Here's the drawing with two shaded views (mm, measured from the low corner). I have some questions. A direction names the side the tool comes from. Round coordinates to 2 decimals unless told otherwise and drop trailing zeros. Write each loop counter-clockwise with the first axis right and the second up, starting at its lowest first coordinate (ties: lowest second). Pieces come first, ordered by that corner, then holes. Notation, with made-up numbers: M 73.25,3.5 L 127.25,3.5 A34 ccw 127.25,33.5 Z; hole C 75,75.5 d3. An arc over 180 degrees is marked long. Answer as a JSON object with one key per item and string values. Group by question number.
1) Suppose I cut it at A-A, the plane x = 120. Write out the boundary of the cut face in (y, z), and give its area (3 significant figures).
2) Suppose I cut it at C-C, the plane z = 36. Write out the boundary of the cut face in (x, y).
3) I'm going to push flat-ended pins straight in: pin 1 Ø7.5 at (x, y) = (65.5, 120.5) entering from +Z (1 decimal); pin 2 Ø5 at (x, y) = (89.5, 3) entering from +Z; pin 3 Ø17 at (y, z) = (62.12, 48.86) entering from -X. Where does each tip first touch, or does it pass through?
4) If we mould it in two halves opening along X, with no side actions, what happens to the marked faces 3, 4 and 5? For each: +X half, -X half, draft (parallel to the pull), parting line (faces both ways), or undercut.
5) Suppose I cut it at D-D, the plane z = 52. Write out the boundary of the cut face in (x, y).
6) On a 3-axis mill with a long thin cutter (end or side, diameter ignored), from which of +Z, -Z, +X, -X, +Y, -Y can I reach the whole of each face in a straight line? I mean the marked faces 1 and 2. Say none if no direction works.
7) Please list where these lines run through material, in increasing order: L1, parallel to X at y = 51, z = 64; L2, parallel to Y at x = 46, z = 27.5; L3, parallel to X at y = 119, z = 82. Write a range as [from, to].
8) Suppose I cut it at B-B, the plane y = 84. Write out the boundary of the cut face in (x, z), and give its area (3 significant figures).
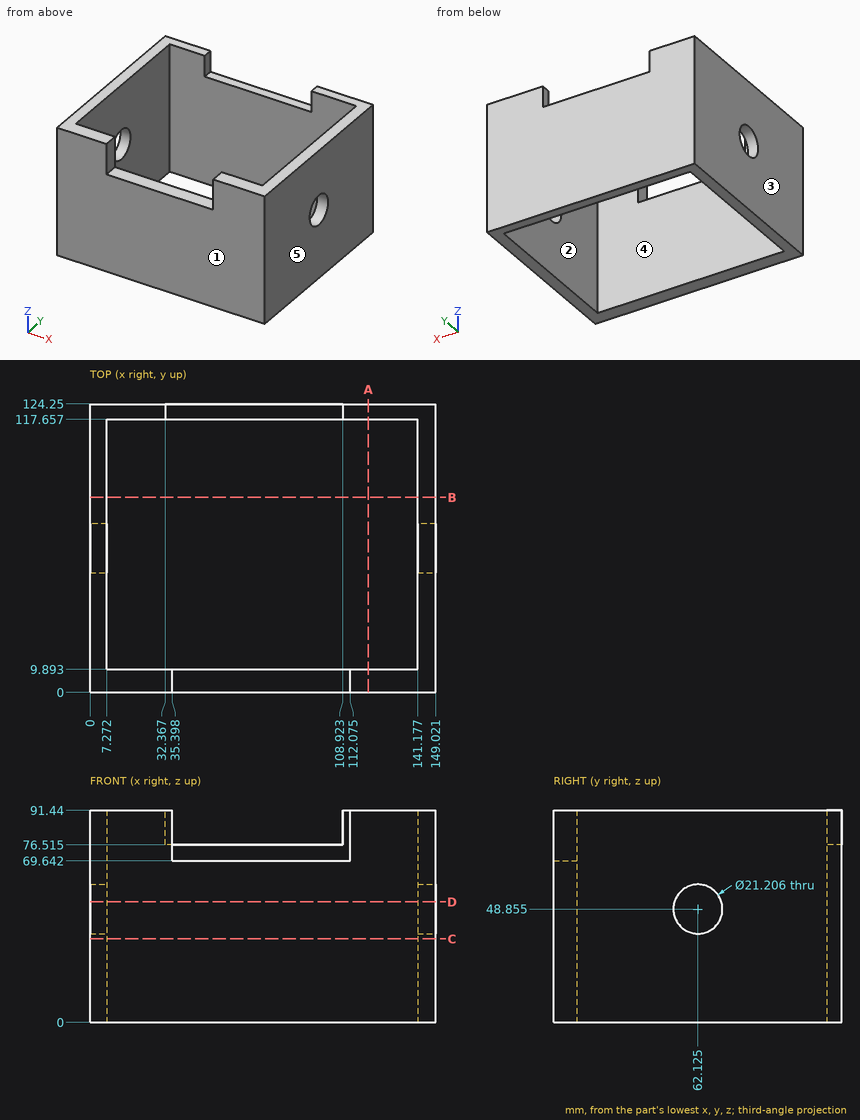
Results:
{
 "1": {"outline": "M 0,0 L 9.89,0 L 9.89,91.44 L 0,91.44 Z; M 117.66,0 L 124.25,0 L 124.25,91.44 L 117.66,91.44 Z", "area": "1,510 mm^2"},
 "2": {"outline": "M 0,0 L 149.02,0 L 149.02,124.25 L 0,124.25 Z; hole M 7.27,9.89 L 141.18,9.89 L 141.18,117.66 L 7.27,117.66 Z"},
 "3": {"pin 1": "z = 76.5", "pin 2": "z = 69.64", "pin 3": "through"},
 "4": {"face 3": "-X half", "face 4": "undercut", "face 5": "+X half"},
 "5": {"outline": "M 0,0 L 149.02,0 L 149.02,52 L 141.18,52 L 141.18,9.89 L 7.27,9.89 L 7.27,52 L 0,52 Z; M 0,72.25 L 7.27,72.25 L 7.27,117.66 L 141.18,117.66 L 141.18,72.25 L 149.02,72.25 L 149.02,124.25 L 0,124.25 Z"},
 "6": {"face 1": "+Z, -Z, +X, -X, -Y", "face 2": "+Z, -Z"},
 "7": {"L1": "[0, 7.27], [141.18, 149.02]", "L2": "[0, 9.89], [117.66, 124.25]", "L3": "[0, 32.37], [108.92, 149.02]"},
 "8": {"outline": "M 0,0 L 7.27,0 L 7.27,91.44 L 0,91.44 Z; M 141.18,0 L 149.02,0 L 149.02,91.44 L 141.18,91.44 Z", "area": "1,380 mm^2"}
}
